from build123d import *

# Parameters (mm, degrees)
SKETCH1_W           = 125
SKETCH1_H           = 45
BOSS_EXTRUDE1_DEPTH = 2
SKETCH2_R           = 2.25
CUT_EXTRUDE1_DEPTH  = 10
SKETCH3_R           = 1.7
CUT_EXTRUDE2_DEPTH  = 10
SKETCH4_W           = 40
SKETCH4_H           = 6
CUT_EXTRUDE3_DEPTH  = 10


with BuildPart() as part:
    # Sketch1 → Boss-Extrude1 (new body)
    with BuildSketch(Plane(origin=(0, 0, 0), x_dir=(1, 0, 0), z_dir=(0, 1, 0))):
        Rectangle(SKETCH1_W, SKETCH1_H)
    extrude(amount=BOSS_EXTRUDE1_DEPTH)

    # Sketch2 → Cut-Extrude1 (cut)
    with BuildSketch(Plane(origin=(0, 2, 0), x_dir=(1, 0, 0), z_dir=(0, 1, 0))):
        with Locations((-10, -12.5)):
            Circle(SKETCH2_R)
        with Locations((10, -12.5)):
            Circle(SKETCH2_R)
        with Locations((-10, 7.5)):
            Circle(SKETCH2_R)
        with Locations((10, 7.5)):
            Circle(SKETCH2_R)
    extrude(amount=-CUT_EXTRUDE1_DEPTH, mode=Mode.SUBTRACT)

    # Sketch3 → Cut-Extrude2 (cut)
    with BuildSketch(Plane(origin=(0, 2, 0), x_dir=(1, 0, 0), z_dir=(0, 1, 0))):
        with Locations((57.5, -7.5)):
            Circle(SKETCH3_R)
        with Locations((35.5, -7.5)):
            Circle(SKETCH3_R)
        with Locations((-35.504729394, -7.5)):
            Circle(SKETCH3_R)
        with Locations((-57.5, -7.5)):
            Circle(SKETCH3_R)
    extrude(amount=-CUT_EXTRUDE2_DEPTH, mode=Mode.SUBTRACT)

    # Sketch4 → Cut-Extrude3 (cut)
    with BuildSketch(Plane(origin=(0, 2, 0), x_dir=(1, 0, 0), z_dir=(0, 1, 0))):
        with Locations((0, 19.5)):
            Rectangle(SKETCH4_W, SKETCH4_H)
    extrude(amount=-CUT_EXTRUDE3_DEPTH, mode=Mode.SUBTRACT)


solid = part.part
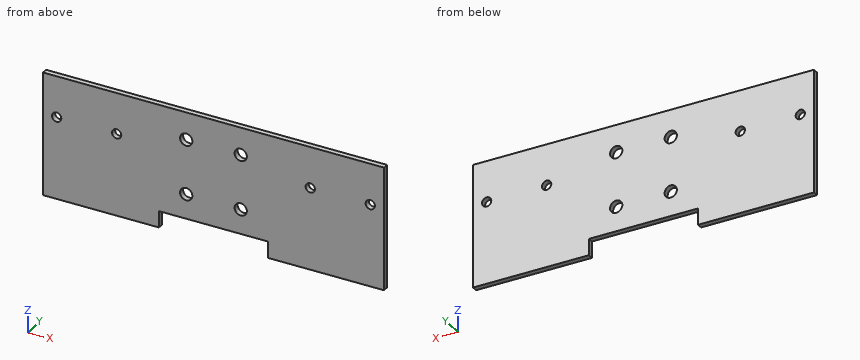
The model under review builds one solid part; all positions refer to its coordinate system, in mm. Round coordinates to 2 decimals unless told otherwise and drop trailing zeros. Loops run counter-clockwise (first coordinate to the right, second up) from the corner with the lowest first, then second, coordinate; pieces in that order, holes last. Notation, with made-up numbers: M 71.25,14.25 L 106.25,14.25 A27 ccw 106.25,51.25 Z; hole C 65,-33 d2. An arc over 180 degrees is marked long. Answer as CSV lines item,"result".
1. To check wall thickness, follow L1, parallel to X at y = 0.65, z = 7.5; L2, parallel to X at y = 0.9, z = -7.5; L3, parallel to Z at x = 10, y = 0.65. State the ranges of each line that lie inside material, in increasing order. Write a range as [from, to].
Outcome:
L1,"x = [-62.5, -59.2], [-55.8, -37.2], [-33.8, 33.8], [37.2, 55.8], [59.2, 62.5]"
L2,"x = [-62.5, -12.25], [-7.75, 7.75], [12.25, 62.5]"
L3,"z = [-16.5, -9.75], [-5.25, 10.25], [14.75, 22.5]"
2. We need section C-C (x = 10). Give the boundary of the cut face in (y, z).
Outcome:
outline,"M 0,-16.5 L 2,-16.5 L 2,-9.75 L 0,-9.75 Z; M 0,-5.25 L 2,-5.25 L 2,10.25 L 0,10.25 Z; M 0,14.75 L 2,14.75 L 2,22.5 L 0,22.5 Z"
3. We need section A-A (x = 35.5). Give the boundary of the cut face in (y, z).
Outcome:
outline,"M 0,-22.5 L 2,-22.5 L 2,5.8 L 0,5.8 Z; M 0,9.2 L 2,9.2 L 2,22.5 L 0,22.5 Z"
4. We need section B-B (z = -7.5). Give the boundary of the cut face in (x, y).
Outcome:
outline,"M -62.5,0 L -12.25,0 L -12.25,2 L -62.5,2 Z; M -7.75,0 L 7.75,0 L 7.75,2 L -7.75,2 Z; M 12.25,0 L 62.5,0 L 62.5,2 L 12.25,2 Z"
5. We need section D-D (y = 0.6). Count the separate pieces of the cut face and the enclosed holes in it, plus the area to 3 significant figures.
Outcome:
separate pieces,"1"
enclosed holes,"8"
area,"5,290 mm2"
6. Insertion check: pin 1 Ø5 at (x, z) = (31, -4.5) entering from -Y; pin 2 Ø2 at (x, z) = (57.5, 7.5) entering from -Y; pin 3 Ø1 at (x, y) = (-3.5, 0.5) entering from -Z. Each pin has a flat end and moves straight along its axis. Give the tip position at first contact, or say it passes through.
Outcome:
pin 1,"stops at y = 0"
pin 2,"passes through"
pin 3,"stops at z = -16.5"
